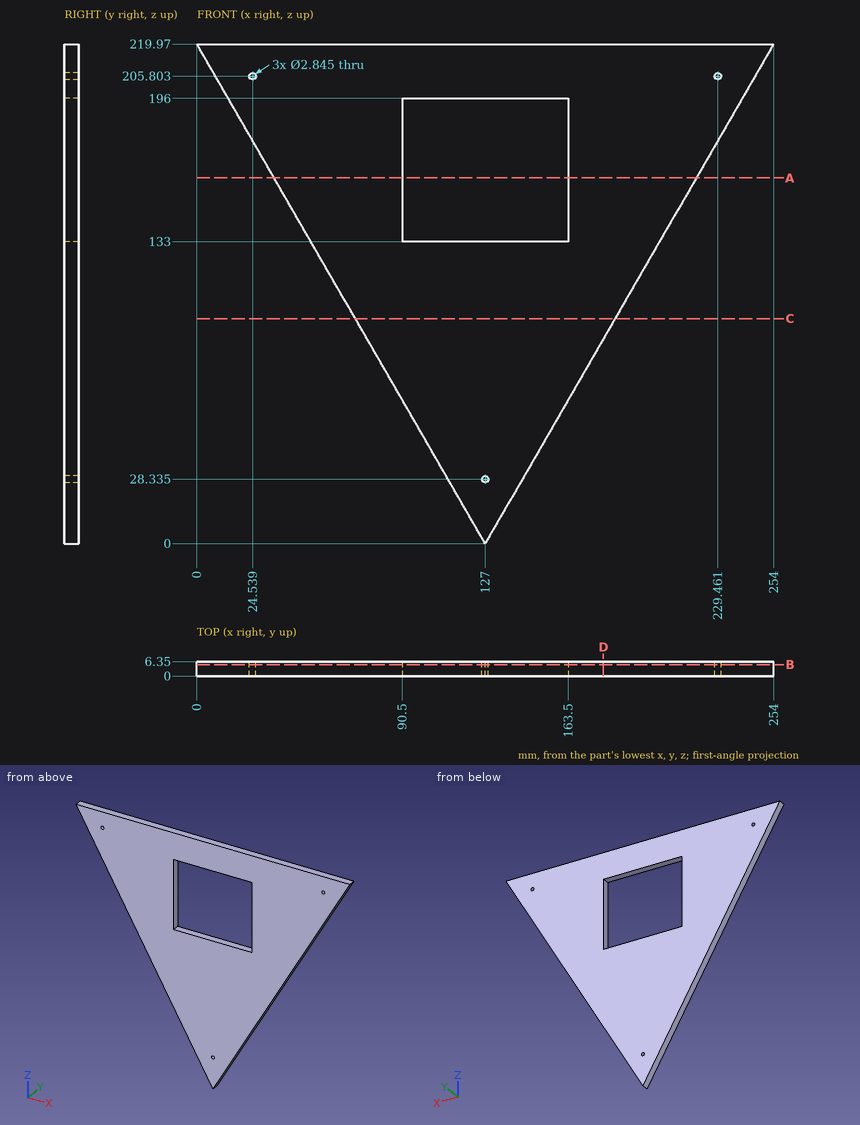
Can you work these out from the drawing? Everything is in mm from the part's minimum corner. Round coordinates to 2 decimals unless told otherwise and drop trailing zeros. Loops run counter-clockwise (first coordinate to the right, second up) from the corner with the lowest first, then second, coordinate; pieces in that order, holes last. Notation, with made-up numbers: (2.25, -15.5) - (32.25, -15.5) arc R34 cw to (32.25, 14.5) - close; hole circle Ø7 at (7.25, -19.5). An arc over 180 degrees is marked (long way). Answer in a Markdown table with one row per item. Add a question column.
Q1. I need wall thicknesses on L1, parallel to Z at x = 127, y = 2.25 (1 decimal); L2, parallel to X at y = 5.25, z = 134 (1 decimal); L3, parallel to Z at x = 127.5, y = 5 (1 decimal). Which ranges of each line are inside material? Lowest first, please.
Q2. I want a section at A-A on z = 161. List the corners of the cut face in (x, y) for me, and give its area (3 significant figures).
Q3. For pin 1 Ø3 at (x, y) = (27.5, 3) entering from -Z; pin 2 Ø1 at (y, z) = (3, 102.5) entering from -X, each with a flat end and sliding along its axis, tell me the tip position at first contact or that it passes through.
Q4. I want a section at D-D on x = 179. List the corners of the cut face in (y, z) for me, and give its area (3 significant figures).
Q5. I want a section at B-B on y = 5. List the corners of the cut face in (x, z) for me (1 decimal), and give its area (3 significant figures).
Q6. I want a section at C-C on z = 99. List the corners of the cut face in (x, y) for me.
A:
| question | item | result |
|---|---|---|
| 1 | L1 | 0 to 26.9, 29.8 to 133, 196 to 220 |
| 1 | L2 | 49.6 to 90.5, 163.5 to 204.4 |
| 1 | L3 | 0.9 to 27, 29.7 to 133, 196 to 220 |
| 2 | outline | (34.05, 0) - (90.5, 0) - (90.5, 6.35) - (34.05, 6.35) - close; (163.5, 0) - (219.95, 0) - (219.95, 6.35) - (163.5, 6.35) - close |
| 2 | area | 717 mm^2 |
| 3 | pin 1 | z = 169.74 |
| 3 | pin 2 | x = 67.53 |
| 4 | outline | (0, 90.07) - (6.35, 90.07) - (6.35, 219.97) - (0, 219.97) - close |
| 4 | area | 825 mm^2 |
| 5 | outline | (0, 220) - (127, 0) - (254, 220) - close; hole circle Ø2.8 at (24.5, 205.8); hole (90.5, 133) - (163.5, 133) - (163.5, 196) - (90.5, 196) - close; hole circle Ø2.8 at (127, 28.3); hole circle Ø2.8 at (229.5, 205.8) |
| 5 | area | 23,300 mm^2 |
| 6 | outline | (69.84, 0) - (184.16, 0) - (184.16, 6.35) - (69.84, 6.35) - close |
